Verification items for the finished model (mm, model axes). Give positions to 0.01 mm unless a question says otherwise; leave off trailing zeros. Loops run counter-clockwise (first coordinate to the right, second up) from the corner with the lowest first, then second, coordinate; pieces in that order, holes last. Notation, with made-up numbers: (66, 40.25) -> (93, 40.25) arc R21 ccw to (93, 79.25) -> close; hole circle Ø9 at (-4.5, -18.75). An arc over 180 degrees is marked (long way). Answer in a Markdown table with one row per item. Add a question column.
Q1. Material ranges on probe 1 along X at (y, z) = (27, 1.5); probe 2 along Y at (x, z) = (21.5, 0.4); probe 3 along X at (y, z) = (46.5, 0.9), recorded low to high.
Q2. Section check B-B on x = 5.5. Give the number of separate pieces and of enclosed holes in the cut face, and give its area (3 significant figures).
Q3. Section check A-A on x = 38. Enter the section's corners in (y, z), and give its area (3 significant figures).
```python
from build123d import *

# Parameters (mm, degrees)
F0_W     = 55.88
F0_H     = 86.36
F0_R     = 1.778
F0_R_2   = 6.35
F0_R_3   = 2.130313
F1_DEPTH = 2.032


with BuildPart() as f1:
    # F0 (on Top) → F1 (new body)
    with BuildSketch(Plane.XY):
        with Locations((27.94, 43.18)):
            Rectangle(F0_W, F0_H)
        with Locations((5.08, 13.716)):
            Circle(F0_R, mode=Mode.SUBTRACT)
        with Locations((11.6332, 15.0368)):
            Circle(F0_R, mode=Mode.SUBTRACT)
        with Locations((11.6332, 20.2692)):
            Circle(F0_R, mode=Mode.SUBTRACT)
        with Locations((18.542, 17.399)):
            Circle(F0_R, mode=Mode.SUBTRACT)
        with Locations((25.4508, 15.0368)):
            Circle(F0_R, mode=Mode.SUBTRACT)
        with Locations((25.4508, 20.2692)):
            Circle(F0_R, mode=Mode.SUBTRACT)
        with Locations((5.08, 21.59)):
            Circle(F0_R, mode=Mode.SUBTRACT)
        with Locations((8.763, 27.178)):
            Circle(F0_R, mode=Mode.SUBTRACT)
        with Locations((5.08, 32.766)):
            Circle(F0_R, mode=Mode.SUBTRACT)
        with Locations((5.08, 40.64)):
            Circle(F0_R, mode=Mode.SUBTRACT)
        with Locations((11.6332, 34.0868)):
            Circle(F0_R, mode=Mode.SUBTRACT)
        with Locations((11.6332, 39.3192)):
            Circle(F0_R, mode=Mode.SUBTRACT)
        with Locations((18.542, 27.178)):
            Circle(F0_R_2, mode=Mode.SUBTRACT)
        with Locations((18.542, 36.957)):
            Circle(F0_R, mode=Mode.SUBTRACT)
        with Locations((25.4508, 34.0868)):
            Circle(F0_R, mode=Mode.SUBTRACT)
        with Locations((25.4508, 39.3192)):
            Circle(F0_R, mode=Mode.SUBTRACT)
        with Locations((32.004, 13.716)):
            Circle(F0_R, mode=Mode.SUBTRACT)
        with Locations((43.18, 13.716)):
            Circle(F0_R, mode=Mode.SUBTRACT)
        with Locations((49.7332, 15.0368)):
            Circle(F0_R, mode=Mode.SUBTRACT)
        with Locations((49.7332, 20.2692)):
            Circle(F0_R, mode=Mode.SUBTRACT)
        with Locations((32.004, 21.59)):
            Circle(F0_R, mode=Mode.SUBTRACT)
        with Locations((28.321, 27.178)):
            Circle(F0_R, mode=Mode.SUBTRACT)
        with Locations((32.004, 32.766)):
            Circle(F0_R, mode=Mode.SUBTRACT)
        with Locations((32.004, 40.64)):
            Circle(F0_R, mode=Mode.SUBTRACT)
        with Locations((43.18, 21.59)):
            Circle(F0_R, mode=Mode.SUBTRACT)
        with Locations((46.863, 27.178)):
            Circle(F0_R, mode=Mode.SUBTRACT)
        with Locations((43.18, 32.766)):
            Circle(F0_R, mode=Mode.SUBTRACT)
        with Locations((43.18, 40.64)):
            Circle(F0_R, mode=Mode.SUBTRACT)
        with Locations((49.7332, 34.0868)):
            Circle(F0_R, mode=Mode.SUBTRACT)
        with Locations((49.7332, 39.3192)):
            Circle(F0_R, mode=Mode.SUBTRACT)
        with Locations((5.08, 51.816)):
            Circle(F0_R, mode=Mode.SUBTRACT)
        with Locations((11.6332, 53.1368)):
            Circle(F0_R, mode=Mode.SUBTRACT)
        with Locations((5.08, 59.69)):
            Circle(F0_R, mode=Mode.SUBTRACT)
        with Locations((11.6332, 58.3692)):
            Circle(F0_R, mode=Mode.SUBTRACT)
        with Locations((25.4508, 53.1368)):
            Circle(F0_R, mode=Mode.SUBTRACT)
        with Locations((18.542, 55.499)):
            Circle(F0_R, mode=Mode.SUBTRACT)
        with Locations((25.4508, 58.3692)):
            Circle(F0_R, mode=Mode.SUBTRACT)
        with Locations((5.08, 70.866)):
            Circle(F0_R, mode=Mode.SUBTRACT)
        with Locations((8.763, 65.278)):
            Circle(F0_R, mode=Mode.SUBTRACT)
        with Locations((11.6332, 72.1868)):
            Circle(F0_R, mode=Mode.SUBTRACT)
        with Locations((5.08, 78.74)):
            Circle(F0_R, mode=Mode.SUBTRACT)
        with Locations((11.6332, 77.4192)):
            Circle(F0_R, mode=Mode.SUBTRACT)
        with Locations((18.542, 65.278)):
            Circle(F0_R_2, mode=Mode.SUBTRACT)
        with Locations((18.542, 75.057)):
            Circle(F0_R, mode=Mode.SUBTRACT)
        with Locations((25.4508, 72.1868)):
            Circle(F0_R, mode=Mode.SUBTRACT)
        with Locations((25.4508, 77.4192)):
            Circle(F0_R, mode=Mode.SUBTRACT)
        with Locations((32.004, 51.816)):
            Circle(F0_R, mode=Mode.SUBTRACT)
        with Locations((37.084, 46.228)):
            Circle(F0_R_3, mode=Mode.SUBTRACT)
        with Locations((32.004, 59.69)):
            Circle(F0_R, mode=Mode.SUBTRACT)
        with Locations((43.18, 51.816)):
            Circle(F0_R, mode=Mode.SUBTRACT)
        with Locations((49.7332, 53.1368)):
            Circle(F0_R, mode=Mode.SUBTRACT)
        with Locations((43.18, 59.69)):
            Circle(F0_R, mode=Mode.SUBTRACT)
        with Locations((49.7332, 58.3692)):
            Circle(F0_R, mode=Mode.SUBTRACT)
        with Locations((28.321, 65.278)):
            Circle(F0_R, mode=Mode.SUBTRACT)
        with Locations((32.004, 70.866)):
            Circle(F0_R, mode=Mode.SUBTRACT)
        with Locations((32.004, 78.74)):
            Circle(F0_R, mode=Mode.SUBTRACT)
        with Locations((46.863, 65.278)):
            Circle(F0_R, mode=Mode.SUBTRACT)
        with Locations((43.18, 70.866)):
            Circle(F0_R, mode=Mode.SUBTRACT)
        with Locations((49.7332, 72.1868)):
            Circle(F0_R, mode=Mode.SUBTRACT)
        with Locations((43.18, 78.74)):
            Circle(F0_R, mode=Mode.SUBTRACT)
        with Locations((49.7332, 77.4192)):
            Circle(F0_R, mode=Mode.SUBTRACT)
    extrude(amount=F1_DEPTH)


solid = f1.part
```
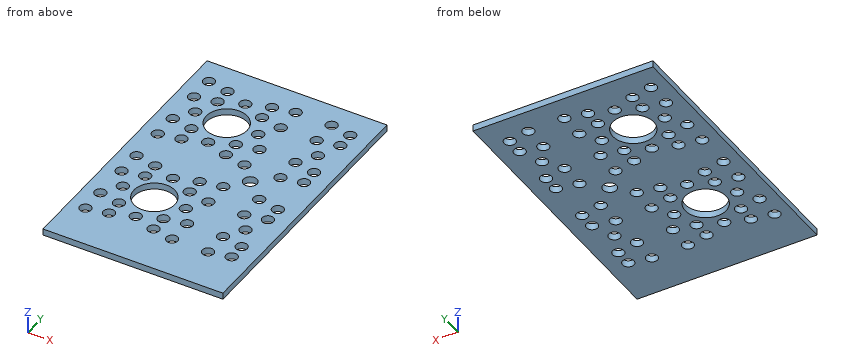
Taken from the geometry:
| question | item | result |
|---|---|---|
| 1 | probe 1 | x = 0 to 6.99, 10.53 to 12.19, 24.89 to 26.55, 30.09 to 45.09, 48.63 to 55.88 |
| 1 | probe 2 | y = 0 to 21.56, 32.8 to 59.66, 70.9 to 86.36 |
| 1 | probe 3 | x = 0 to 34.97, 39.2 to 55.88 |
| 2 | separate pieces | 9 |
| 2 | enclosed holes | 0 |
| 2 | area | 119 mm² |
| 3 | outline | (0, 0) -> (44.3, 0) -> (44.3, 2.03) -> (0, 2.03) -> close; (48.15, 0) -> (86.36, 0) -> (86.36, 2.03) -> (48.15, 2.03) -> close |
| 3 | area | 168 mm² |
